from build123d import *

# Parameters (mm, degrees)
F1_DEPTH = 12.44
F3_DEPTH = 2.28
F4_R     = 1
F5_DEPTH = 1.42


with BuildPart() as f1:
    # F0 (on Top) → F1 (new body, symmetric)
    with BuildSketch(Plane.XY):
        with BuildLine():
            Line((-7.3253149017, -7), (7.3253149017, -7))
            ThreePointArc((7.3253149017, -7), (8.7137955042, -3.6216957288), (9.1872278446, 0))
            ThreePointArc((9.1872278446, 0), (8.7137955042, 3.6216957288), (7.3253149017, 7))
            Line((7.3253149017, 7), (-7.3253149017, 7))
            ThreePointArc((-7.3253149017, 7), (-8.7137955052, 3.6216957251), (-9.1872278446, -7.5e-09))
            ThreePointArc((-9.1872278446, -7.5e-09), (-8.7137955032, -3.6216957324), (-7.3253149017, -7))
        make_face()
    extrude(amount=F1_DEPTH, both=True)

    # F2 (on face) → F3 (join)
    with BuildSketch(Plane(origin=(0, 0, -12.44), x_dir=(1, 0, 0), z_dir=(0, 0, -1))):
        with BuildLine():
            ThreePointArc((3.0027986946, -3.91), (4.4220299391, -2.1795759262), (4.93, 0))
            ThreePointArc((4.93, 0), (-2.1795759262, 4.4220299391), (-3.0027986946, -3.91))
            Line((-3.0027986946, -3.91), (3.0027986946, -3.91))
        make_face()
    extrude(amount=F3_DEPTH)

    # F4 (on face) → F5 (join)
    with BuildSketch(Plane(origin=(0, 0, -14.72), x_dir=(1, 0, 0), z_dir=(0, 0, -1))):
        Circle(F4_R)
    extrude(amount=F5_DEPTH)


solid = f1.part
Here's how the part is built. I have some questions about the finished solid (model axes, mm). A direction names the side the tool comes from. Coordinates: 2 decimals unless noted, no trailing zeros. Order: outer loops, then holes, each group sorted by start corner. A loop starts at its lowest first (then second) coordinate and runs counter-clockwise, first axis right, second up. Notation, with made-up numbers: M -31.5,43.25 L 22.5,43.25 A12 ccw 22.5,50.25 Z; hole C 82,-40 d5. An arc over 180 degrees is marked long. Answer as CSV lines item,"result". Start each with the question number.
1. I want a section at B-B, the plane y = 1.75. Write out the boundary of the cut face in (x, z), and give its area (3 significant figures).
2. I want a section at A-A, the plane x = 0. Write out the boundary of the cut face in (y, z), and give its area (3 significant figures).
3. For pin 1 (2.5 mm diameter, centred on x = 1.5, z = -14, fed in from +Y); pin 2 (1.5 mm diameter, centred on x = -5.5, y = 4, fed in from -Z); pin 3 (1.5 mm diameter, centred on y = 3, z = -11.5, fed in from +X), each with a flat end and sliding along its axis, tell me the tip position at first contact or that it passes through.
4. I need wall thicknesses on line 1 (Z direction, x = -8, y = 2); line 2 (Z direction, x = -2.5, y = -2.5); line 3 (X direction, y = 5.5, z = -10.25). Which ranges of each line are inside material? Lowest first, please. Write a range as [from, to].
5. I want a section at D-D, the plane x = 3.5. Write out the boundary of the cut face in (y, z).
6. On a 3-axis mill with a long thin cutter (end or side, diameter ignored), from which of +Z, -Z, +X, -X, +Y, -Y can I reach the whole of each face in a straight line? I mean faces 1 (the flat face through (0, 0, 12.44)), 2 (the flat face through (0, 5, -12.44)), 3 (the flat face through (0, 3.91, -14)). Say none if no direction works.
7. I want a section at C-C, the plane z = -0.5. Write out the boundary of the cut face in (x, y).
Recorded:
1,outline,"M -9.08,-12.44 L -4.61,-12.44 L -4.61,-14.72 L 4.61,-14.72 L 4.61,-12.44 L 9.08,-12.44 L 9.08,12.44 L -9.08,12.44 Z"
1,area,"473 mm2"
2,outline,"M -7,-12.44 L -4.93,-12.44 L -4.93,-14.72 L -1,-14.72 L -1,-16.14 L 1,-16.14 L 1,-14.72 L 3.91,-14.72 L 3.91,-12.44 L 7,-12.44 L 7,12.44 L -7,12.44 Z"
2,area,"371 mm2"
3,pin 1,"stops at y = 3.91"
3,pin 2,"stops at z = -12.44"
3,pin 3,"stops at x = 9.01"
4,line 1,"z = [-12.44, 12.44]"
4,line 2,"z = [-14.72, 12.44]"
4,line 3,"x = [-8.07, 8.07]"
5,outline,"M -7,-12.44 L -3.47,-12.44 L -3.47,-14.72 L 3.47,-14.72 L 3.47,-12.44 L 7,-12.44 L 7,12.44 L -7,12.44 Z"
6,face 1,"+Z, +X, -X, +Y, -Y"
6,face 2,"-Z"
6,face 3,"-Z, +X, -X, +Y"
7,outline,"M -7.33,-7 L 7.33,-7 A14.09 ccw 7.33,7 L -7.33,7 A14.09 ccw Z"
